CAD build for the part. Positions are in the model's coordinates, mm. Round coordinates to 2 decimals unless told otherwise and drop trailing zeros. Loops run counter-clockwise (first coordinate to the right, second up) from the corner with the lowest first, then second, coordinate; pieces in that order, holes last.
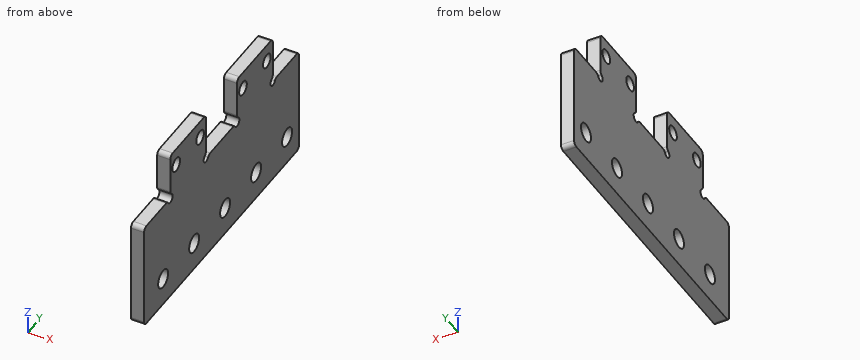
```python
from build123d import *

# Parameters (mm, degrees)
SKETCH_1_W          = 28
SKETCH_1_H          = 65
EXTRUDE_1_DEPTH     = 3
SKETCH_2_W          = 3
SKETCH_2_H          = 11
SKETCH_2_H_2        = 13
CUT_EXTRUDE_1_DEPTH = 71.837842994
SKETCH_3_R          = 2.1
CUT_EXTRUDE_2_DEPTH = 71.837842994
SKETCH_4_R          = 1
CUT_EXTRUDE_3_DEPTH = 71.837842994
SKETCH_5_W          = 3
SKETCH_5_H          = 15
EXTRUDE_2_DEPTH     = 8
SKETCH_6_R          = 1.6
CUT_EXTRUDE_4_DEPTH = 10
FILLET_1_R          = 1


with BuildPart() as part:
    # 草图1 → 凸台-拉伸1 (new body)
    with BuildSketch(Plane(origin=(0, 0, 0), x_dir=(0, 0, -1), z_dir=(1, 0, 0))):
        with Locations((14, 32.5)):
            Rectangle(SKETCH_1_W, SKETCH_1_H)
    extrude(amount=EXTRUDE_1_DEPTH)

    # 草图2 → 切除-拉伸1 (cut, through all)
    with BuildSketch(Plane(origin=(3, 0, 0), x_dir=(0, 0, -1), z_dir=(1, 0, 0))):
        with Locations((1.5, 59.5)):
            Rectangle(SKETCH_2_W, SKETCH_2_H)
        with Locations((1.5, 32.5)):
            Rectangle(SKETCH_2_W, SKETCH_2_H_2)
        with Locations((1.5, 5.5)):
            Rectangle(SKETCH_2_W, SKETCH_2_H)
    extrude(amount=-CUT_EXTRUDE_1_DEPTH, mode=Mode.SUBTRACT)

    # 草图3 → 切除-拉伸2 (cut, through all)
    with BuildSketch(Plane(origin=(3, 0, 0), x_dir=(0, 0, -1), z_dir=(1, 0, 0))):
        with Locations((21.5, 60)):
            Circle(SKETCH_3_R)
        with Locations((21.5, 47)):
            Circle(SKETCH_3_R)
        with Locations((21.5, 34)):
            Circle(SKETCH_3_R)
        with Locations((21.5, 21)):
            Circle(SKETCH_3_R)
        with Locations((21.5, 8)):
            Circle(SKETCH_3_R)
    extrude(amount=-CUT_EXTRUDE_2_DEPTH, mode=Mode.SUBTRACT)

    # 草图4 → 切除-拉伸3 (cut, through all)
    with BuildSketch(Plane(origin=(3, 0, 0), x_dir=(0, 0, -1), z_dir=(1, 0, 0))):
        with Locations((3, 54)):
            Circle(SKETCH_4_R)
        with Locations((3, 39)):
            Circle(SKETCH_4_R)
        with Locations((3, 26)):
            Circle(SKETCH_4_R)
        with Locations((3, 11)):
            Circle(SKETCH_4_R)
    extrude(amount=-CUT_EXTRUDE_3_DEPTH, mode=Mode.SUBTRACT)

    # 草图5 → 凸台-拉伸2 (add)
    with BuildSketch(Plane.XY):
        with Locations((1.5, 18.5)):
            Rectangle(SKETCH_5_W, SKETCH_5_H)
        with Locations((1.5, 46.5)):
            Rectangle(SKETCH_5_W, SKETCH_5_H)
    extrude(amount=EXTRUDE_2_DEPTH)

    # 草图6 → 切除-拉伸4 (cut)
    with BuildSketch(Plane(origin=(3, 0, 0), x_dir=(0, 0, -1), z_dir=(1, 0, 0))):
        with Locations((-4, 51.5)):
            Circle(SKETCH_6_R)
        with Locations((-4, 41.5)):
            Circle(SKETCH_6_R)
        with Locations((-4, 23.5)):
            Circle(SKETCH_6_R)
        with Locations((-4, 13.5)):
            Circle(SKETCH_6_R)
    extrude(amount=-CUT_EXTRUDE_4_DEPTH, mode=Mode.SUBTRACT)

    # 圆角1
    fillet_1_edges = [part.edges().sort_by_distance(p)[0] for p in [
        (1.5, 39, -2),
        (1.5, 27, -3),
        (1.5, 11, -2),
        (1.5, 11, 8),
        (1.5, 26, 8),
        (1.5, 39, 8),
        (1.5, 54, 8),
        (1.5, 65, -3),
        (1.5, 0, -3),
        (1.5, 65, -28),
        (1.5, 0, -28),
        (1.5, 54, -2),
        (1.5, 26, -2),
        (1.5, 38, -3),
        (1.5, 10, -3),
        (1.5, 55, -3),
    ]]
    fillet(fillet_1_edges, radius=FILLET_1_R)


solid = part.part
```
Item 1: Flat gauge pins, fed straight in: P1, Ø1.5, axis at x = 1.5, y = 34, coming from the +Z side; P2, Ø1, axis at x = 2, z = 4, coming from the +Y side; P3, Ø4, axis at y = 8, z = -21.5, coming from the -X side. Where does each tip first touch, or does it go through?
Answers follow:
P1: stops at z = -3
P2: stops at y = 54
P3: passes through
Item 2: Probe line 1 (Y direction, x = 2.35, z = 4); line 2 (Y direction, x = 2.2, z = -21.5); line 3 (Z direction, x = 1.45, y = 29). List the from-to ranges inside material, lowest first.
Answers follow:
line 1: y = 11 to 11.9, 15.1 to 21.9, 25.1 to 26, 39 to 39.9, 43.1 to 49.9, 53.1 to 54
line 2: y = 0 to 5.9, 10.1 to 18.9, 23.1 to 31.9, 36.1 to 44.9, 49.1 to 57.9, 62.1 to 65
line 3: z = -28 to -3
Item 3: Cut at C-C, the plane x = 2.4. State how many separate pieces and enclosed holes the cut face has, plus the area to 3 significant figures.
Answers follow:
separate pieces: 1
enclosed holes: 9
area: 1,840 mm2
Item 4: Cut at B-B, the plane z = -21.5. Give the cut face in (x, y).
Answers follow:
outline: (0, 0) - (3, 0) - (3, 5.9) - (0, 5.9) - close; (0, 10.1) - (3, 10.1) - (3, 18.9) - (0, 18.9) - close; (0, 23.1) - (3, 23.1) - (3, 31.9) - (0, 31.9) - close; (0, 36.1) - (3, 36.1) - (3, 44.9) - (0, 44.9) - close; (0, 49.1) - (3, 49.1) - (3, 57.9) - (0, 57.9) - close; (0, 62.1) - (3, 62.1) - (3, 65) - (0, 65) - close
Item 5: Cut at A-A, the plane y = 51.5. Give the cut face in (x, z).
Answers follow:
outline: (0, -28) - (3, -28) - (3, 2.4) - (0, 2.4) - close; (0, 5.6) - (3, 5.6) - (3, 8) - (0, 8) - close
